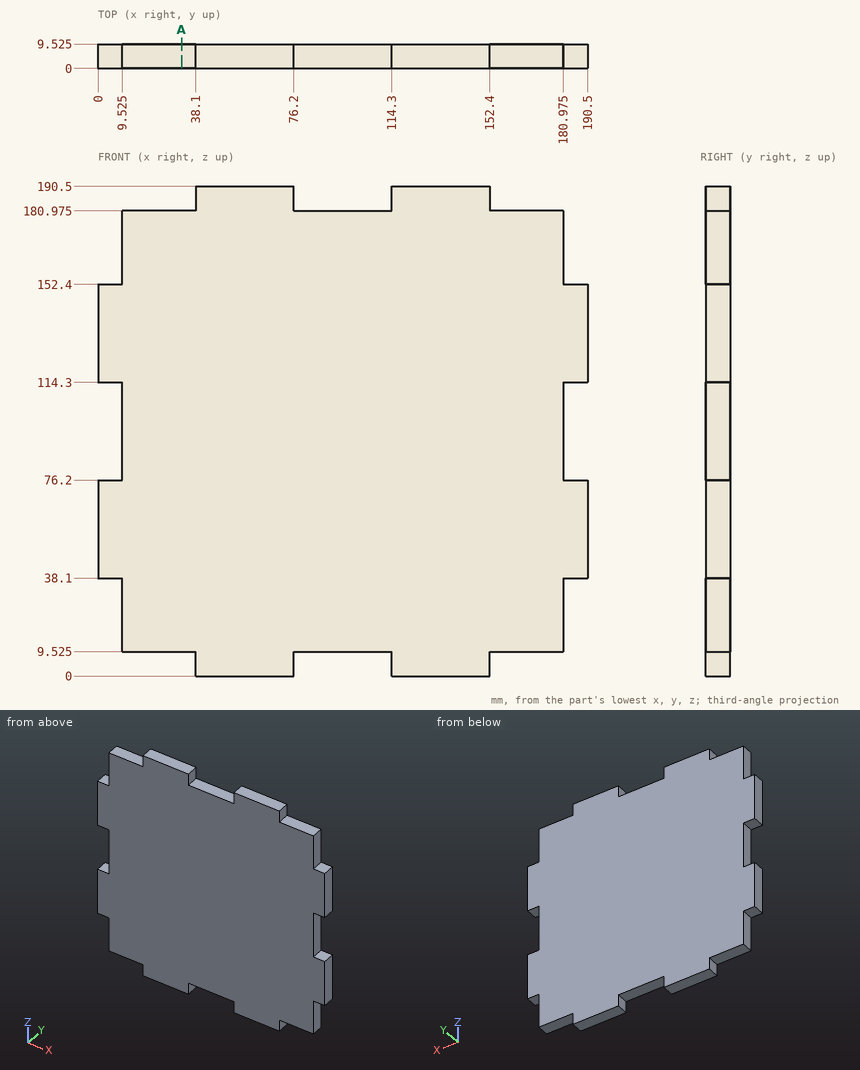
Geometry check sheet. Reference: drawing and pictorial views, mm from the part's lowest x, y, z. Coordinates: 2 decimals unless noted, no trailing zeros. Write each loop counter-clockwise with the first axis right and the second up, starting at its lowest first coordinate (ties: lowest second). Pieces come first, ordered by that corner, then holes. Notation, with made-up numbers: M 47,43 L 52,43 A12 cw 52,62 Z; hole C -2.5,31.5 d3. An arc over 180 degrees is marked long. Write item = value, one per line. Start each with the question number.
1. Sectioned sample at A-A (x = 32.5). Record the cut outline in (y, z) (3 decimals).
2. Thickness scan on probe 1 along X at (y, z) = (3.5, 99) (3 decimals). Record the ranges inside material, lowest first.
3. Go/stop test with flat-tipped pins: pin 1 (5 mm diameter, centred on x = 100, y = 6.5, fed in from -Z) (3 decimals); pin 2 (5 mm diameter, centred on y = 4, z = 3.5, fed in from -X); pin 3 (3 mm diameter, centred on x = 7, y = 5.5, fed in from -Z). Record where each tip stops, or that it passes through.
The answers:
q1.outline = M 0,9.525 L 9.525,9.525 L 9.525,180.975 L 0,180.975 Z
q2.probe_1 = 9.525 to 180.975
q3.pin_1 = 9.525
q3.pin_2 = 38.1
q3.pin_3 = 38.1
